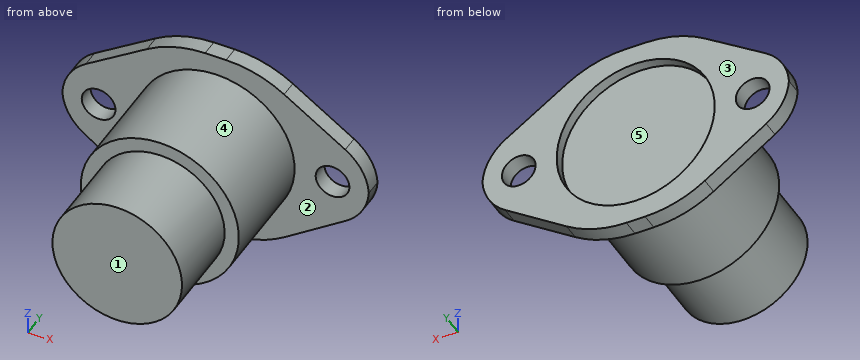
```python
from build123d import *

# Parameters (mm, degrees)
SKETCH1_R           = 7.5
BOSS_EXTRUDE1_DEPTH = 10.2
SKETCH2_R           = 1.6
BOSS_EXTRUDE2_DEPTH = 1.6
SKETCH3_R           = 6.15
BOSS_EXTRUDE3_DEPTH = 7.8
CUT_EXTRUDE1_START  = -1
SKETCH4_R           = 7.5
CUT_EXTRUDE1_DEPTH  = 1
FILLET1_R           = 5
FILLET2_R           = 10


with BuildPart() as part:
    # Sketch1 → Boss-Extrude1 (new body)
    with BuildSketch(Plane(origin=(0, 0, 0), x_dir=(1, 0, 0), z_dir=(0, 1, 0))):
        with Locations(Location((0, 0, 0), (0, 0, 270))):
            Circle(SKETCH1_R)
    extrude(amount=BOSS_EXTRUDE1_DEPTH)

    # Sketch2 → Boss-Extrude2 (add)
    with BuildSketch(Plane(origin=(0, 10.2, 0), x_dir=(1, 0, 0), z_dir=(0, 1, 0))):
        Polygon((-14.55, 2.306992561), (-14.55, -2.466095496), (-4, -9.43480406), (4, -9.43480406), (14.55, -2.466095496), (14.55, 2.306992561), (4, 9.56519594), (-4, 9.56519594), align=None)
        with Locations(Location((-11.1, 0, 0), (0, 0, 270))):
            Circle(SKETCH2_R, mode=Mode.SUBTRACT)
        with Locations(Location((11.1, 0, 0), (0, 0, 270))):
            Circle(SKETCH2_R, mode=Mode.SUBTRACT)
    extrude(amount=BOSS_EXTRUDE2_DEPTH)

    # Sketch3 → Boss-Extrude3 (add)
    with BuildSketch(Plane.XZ):
        with Locations(Location((0, 0, 0), (0, 0, 90))):
            Circle(SKETCH3_R)
    extrude(amount=BOSS_EXTRUDE3_DEPTH)

    # Sketch4 → Cut-Extrude1 (cut)
    with BuildSketch(Plane(origin=(0, 11.8, 0), x_dir=(1, 0, 0), z_dir=(0, 1, 0)).offset(CUT_EXTRUDE1_START)):
        with Locations(Location((0, 0, 0), (0, 0, 270))):
            Circle(SKETCH4_R)
    extrude(amount=CUT_EXTRUDE1_DEPTH, mode=Mode.SUBTRACT)

    # Fillet1
    # the kernel refuses this fillet: 5 mm, written as the material it takes off along each edge
    with BuildSketch(Plane(origin=(14.55, 3.627226277, -2.306992561), x_dir=(-0.8238567421682754, 0, -0.5667980843156368), z_dir=(0, 1, 0)), Plane(origin=(-14.55, 3.627226277, -2.306992561), x_dir=(0, 0, 1), z_dir=(0, 1, 0))) as fillet1_piece_1:
        with BuildLine():
            CenterArc((FILLET1_R * 0.525821897803, FILLET1_R), FILLET1_R, 214.527246886, 55.472753114)
            Line((-FILLET1_R * 0.298034844366, FILLET1_R * 0.433201915684), (0, 0))
            Line((0, 0), (FILLET1_R * 0.525821897803, 0))
        make_face()
    extrude(amount=14.745547445, mode=Mode.SUBTRACT)
    with BuildSketch(Plane(origin=(14.55, 3.475971105, 2.466095496), x_dir=(-0.8344017794446341, 0, 0.5511566659849338), z_dir=(0, 1, 0)), Plane(origin=(-14.55, 3.475971105, 2.466095496), x_dir=(0, 0, -1), z_dir=(0, 1, 0))) as fillet1_piece_2:
        with BuildLine():
            CenterArc((FILLET1_R * 0.537922311616, -FILLET1_R), FILLET1_R, 90, 56.553598673)
            Line((-FILLET1_R * 0.296479467829, -FILLET1_R * 0.448843334015), (0, 0))
            Line((0, 0), (FILLET1_R * 0.537922311616, 0))
        make_face()
    extrude(amount=15.04805779, mode=Mode.SUBTRACT)

    # Fillet2
    fillet2_edges = [part.edges().sort_by_distance(p)[0] for p in [
        (-4, 11, 9.43480406),
        (4, 11, 9.43480406),
        (4, 11, -9.56519594),
        (-4, 11, -9.56519594),
    ]]
    fillet(fillet2_edges, radius=FILLET2_R)


solid = part.part
```
Geometry check sheet. Reference: the model listing, model coordinates, mm. Face numbers are marked on the shaded views. A direction names the side the tool comes from. Coordinates: 2 decimals unless noted, no trailing zeros. Write each loop counter-clockwise with the first axis right and the second up, starting at its lowest first coordinate (ties: lowest second). Pieces come first, ordered by that corner, then holes. Notation, with made-up numbers: M -18,23 L 11,23 A18 cw 11,40 Z; hole C 64,47.25 d10. An arc over 180 degrees is marked long. One line per item, written item: value. Start each with the question number.
(1) Release check for a two-part mould opening along X. For the marked faces 3, 4 and 5 record: released by +X, released by -X, zero draft, split by the parting line, or undercut.
(2) Sectioned sample at A-A, the plane x = 11.1. Enter the section's corners in (y, z).
(3) Sectioned sample at D-D, the plane y = 8.5. Enter the section's corners in (x, z), and give its area (3 significant figures).
(4) Sectioned sample at C-C, the plane z = -2.5. Enter the section's corners in (x, y), and give its area (3 significant figures).
(5) Depth check by flat-ended pin: pin 1 (5 mm diameter, centred on x = 7.5, y = -0.5, fed in from -Z); pin 2 (6 mm diameter, centred on x = -9.5, y = 5, fed in from -Z); pin 3 (5 mm diameter, centred on x = 10, y = -0.5, fed in from -Z) (3 decimals); pin 4 (4 mm diameter, centred on y = -3, z = 1.5, fed in from -X). Enter the tip coordinate at first touch or a pass-through.
(6) Tool access check on the marked faces 1 and 2. Record the directions out of +Z, -Z, +X, -X, +Y, -Y that give a thin tool (end or side, any length) a straight path to the whole face; none if there is none.
(7) Sectioned sample at B-B, the plane x = 0. Enter the section's corners in (y, z), and give its area (3 significant figures).
(8) Scan lines: line 1 along X through (y, z) = (11.1, 0); line 2 along Y through (x, z) = (9.75, 5.5); line 3 along Y through (x, z) = (-4.25, -5.5). Record each from-to range of solid material in increasing order. Write a range as [from, to].
Filled sheet:
1. face 3: zero draft
1. face 4: split by the parting line
1. face 5: undercut
2. outline: M 10.2,-4.68 L 11.8,-4.68 L 11.8,-1.6 L 10.2,-1.6 Z; M 10.2,1.6 L 11.8,1.6 L 11.8,4.74 L 10.2,4.74 Z
3. outline: C 0,0 d15
3. area: 177 mm²
4. outline: M -13.68,10.2 L -7.07,10.2 L -7.07,0 L -5.62,0 L -5.62,-7.8 L 5.62,-7.8 L 5.62,0 L 7.07,0 L 7.07,10.2 L 13.68,10.2 L 13.68,11.8 L 7.07,11.8 L 7.07,10.8 L -7.07,10.8 L -7.07,11.8 L -13.68,11.8 Z
4. area: 262 mm²
5. pin 1: z = -5.54
5. pin 2: z = -3.74
5. pin 3: through
5. pin 4: x = -6.15
6. face 1: +Z, -Z, +X, -X, -Y
6. face 2: -Y
7. outline: M -7.8,-6.15 L 0,-6.15 L 0,-7.5 L 10.2,-7.5 L 10.2,-9.57 L 11.8,-9.57 L 11.8,-7.5 L 10.8,-7.5 L 10.8,7.5 L 11.8,7.5 L 11.8,9.43 L 10.2,9.43 L 10.2,7.5 L 0,7.5 L 0,6.15 L -7.8,6.15 Z
7. area: 264 mm²
8. line 1: [-14.54, -12.7], [-9.5, -7.5], [7.5, 9.5], [12.7, 14.54]
8. line 2: [10.2, 11.8]
8. line 3: [0, 10.8]
